from build123d import *

# Parameters (mm, degrees)
SKETCH1_W           = 88.9
SKETCH1_H           = 41.91
BOSS_EXTRUDE1_DEPTH = 5.08
CUT_EXTRUDE1_REACH  = 93.131
SKETCH2_R           = 2.3495


with BuildPart() as part:
    # Sketch1 → Boss-Extrude1 (new body)
    with BuildSketch(Plane(origin=(0, 0, 0), x_dir=(1, 0, 0), z_dir=(0, 1, 0))):
        with BuildLine():
            ThreePointArc((-77.441755774, -1.121902455), (-85.948469046, -8.106902455), (-77.441755774, -15.091902455))
            Line((-77.441755774, -15.091902455), (-78.827364113, -15.091902455))
            Line((-78.827364113, -15.091902455), (-78.827364113, -1.121902455))
            Line((-78.827364113, -1.121902455), (-77.441755774, -1.121902455))
        make_face()
        with BuildLine():
            Line((-78.827364113, -15.091902455), (-77.441755774, -15.091902455))
            ThreePointArc((-77.441755774, -15.091902455), (-73.323856239, -12.625921878), (-71.70625918, -8.106902455))
            ThreePointArc((-71.70625918, -8.106902455), (-73.323856239, -3.587883032), (-77.441755774, -1.121902455))
            Line((-77.441755774, -1.121902455), (-78.827364113, -1.121902455))
            Line((-78.827364113, -1.121902455), (-78.827364113, -15.091902455))
        make_face()
        with BuildLine():
            Line((-77.441755774, -15.091902455), (-70.953364113, -15.091902455))
            Line((-70.953364113, -15.091902455), (-70.953364113, -1.121902455))
            Line((-70.953364113, -1.121902455), (-77.441755774, -1.121902455))
            ThreePointArc((-77.441755774, -1.121902455), (-73.323856239, -3.587883032), (-71.70625918, -8.106902455))
            ThreePointArc((-71.70625918, -8.106902455), (-73.323856239, -12.625921878), (-77.441755774, -15.091902455))
        make_face()
        with Locations((-26.503364113, -8.911027969)):
            Rectangle(SKETCH1_W, SKETCH1_H)
    boss_extrude1 = extrude(amount=BOSS_EXTRUDE1_DEPTH)

    # Sketch2 → Cut-Extrude1 (cut, up to next)
    with BuildSketch(Plane(origin=(0, 0, 0), x_dir=(-1, 0, 0), z_dir=(0, -1, 0)), mode=Mode.PRIVATE) as cut_extrude1_sk1:
        with Locations(Location((78.827364113, -8.106902455, 0), (0, 0, 90))):
            Circle(SKETCH2_R)
    cut_extrude1_tool1 = extrude(cut_extrude1_sk1.sketch, amount=-CUT_EXTRUDE1_REACH, mode=Mode.PRIVATE) & part.part
    cut_extrude1 = cut_extrude1_tool1.solids().sort_by_distance((-78.827364, 0, 8.106902))[0]
    add(cut_extrude1, mode=Mode.SUBTRACT)

    # Mirror2: Boss-Extrude1, Cut-Extrude1 across plane
    add(boss_extrude1.mirror(Plane(origin=(17.946635887, 5.08, 0), x_dir=(0, 0, 1), z_dir=(-1, 0, 0))))
    add(cut_extrude1.mirror(Plane(origin=(17.946635887, 5.08, 0), x_dir=(0, 0, 1), z_dir=(-1, 0, 0))), mode=Mode.SUBTRACT)


solid = part.part
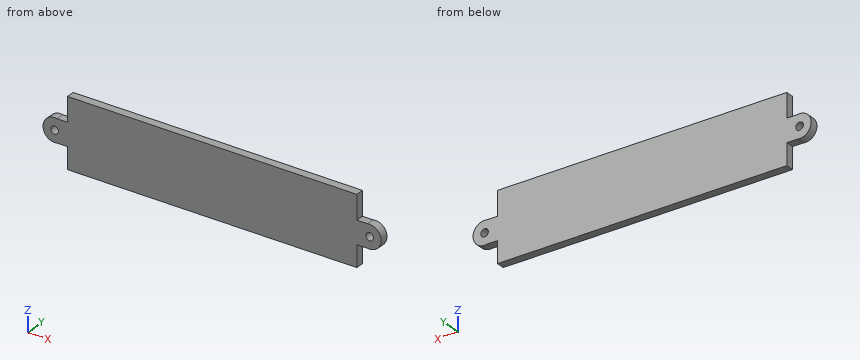
Work out the finished part from the listing and answer in its coordinate system (mm). Round coordinates to 2 decimals unless told otherwise and drop trailing zeros. Order: outer loops, then holes, each group sorted by start corner. A loop starts at its lowest first (then second) coordinate and runs counter-clockwise, first axis right, second up. Notation, with made-up numbers: M 44.25,-31.75 L 58.25,-31.75 A5 ccw 58.25,-26.75 Z; hole C 83,3 d2. An arc over 180 degrees is marked long. Put each result on its own line as item: value. Start each with the question number.
Q1. Section C-C, the plane z = -6 is taken. Write down the section's boundary in (x, y), and give its area (3 significant figures).
Q2. Flat-ended cylindrical pins translate along their axes: pin 1 (5.5 mm diameter, centred on x = 114.72, z = 8.11, fed in from +Y); pin 2 (3 mm diameter, centred on y = 2.5, z = 18, fed in from -X); pin 3 (1.5 mm diameter, centred on y = 1.5, z = -7, fed in from +X); pin 4 (1.5 mm diameter, centred on x = 109, y = 3.5, fed in from -Z). Find the tip coordinate at first contact, or state that the pin passes through.
Q3. Section B-B, the plane y = 1 is taken. Write down the section's boundary in (x, z), and give its area (3 significant figures).
Q4. Section A-A, the plane z = 8.5 is taken. Write down the section's boundary in (x, y).
Q5. Straight lines are drawn through the part: L1, parallel to X at y = 2.7, z = 27; L2, parallel to Z at x = 111.5, y = 4.8; L3, parallel to X at y = 2.9, z = 4.5. For each, find the intervals that lie inside material, in ascending order. Write a range as [from, to].
Findings below:
1. outline: M -70.95,0 L 106.85,0 L 106.85,5.08 L -70.95,5.08 Z
1. area: 903 mm^2
2. pin 1: stops at y = 5.08
2. pin 2: stops at x = -70.95
2. pin 3: stops at x = 106.85
2. pin 4: stops at z = 1.12
3. outline: M -77.44,1.12 L -70.95,1.12 L -70.95,-12.04 L 106.85,-12.04 L 106.85,1.12 L 113.34,1.12 A7.12 ccw long 113.34,15.09 L 106.85,15.09 L 106.85,29.87 L -70.95,29.87 L -70.95,15.09 L -77.44,15.09 A7.12 ccw long Z; hole C -78.83,8.11 d4.7; hole C 114.72,8.11 d4.7
3. area: 7,800 mm^2
4. outline: M -85.94,0 L -81.14,0 L -81.14,5.08 L -85.94,5.08 Z; M -76.51,0 L 112.4,0 L 112.4,5.08 L -76.51,5.08 Z; M 117.04,0 L 121.83,0 L 121.83,5.08 L 117.04,5.08 Z
5. L1: x = [-70.95, 106.85]
5. L2: z = [1.12, 15.09]
5. L3: x = [-84.97, 120.86]
